```python
from build123d import *

# Parameters (mm, degrees)
SKETCH1_W            = 43.08
SKETCH1_H            = 16.08
SKETCH1_W_2          = 38
SKETCH1_H_2          = 11
BOSS_EXTRUDE1_DEPTH  = 57.785
SKETCH1_2_W          = 43.08
SKETCH1_2_H          = 16.08
SKETCH1_2_W_2        = 38
SKETCH1_2_H_2        = 11
BOSS_EXTRUDE2_DEPTH  = 2.54
CUT_EXTRUDE2_DEPTH   = 2.54
SKETCH5_W            = 11.811
SKETCH5_H            = 43.08
BOSS_EXTRUDE8_DEPTH  = 2.54
SKETCH5_6_R          = 1.27
BOSS_EXTRUDE9_DEPTH  = 6.35
SKETCH5_8_R          = 1.896612794
SKETCH5_8_R_2        = 1.27
BOSS_EXTRUDE10_DEPTH = 3.81
SKETCH6_W            = 43.08
SKETCH6_H            = 16.08
BOSS_EXTRUDE11_DEPTH = 3.81
SKETCH7_W            = 43.08
SKETCH7_H            = 2.54
BOSS_EXTRUDE12_DEPTH = 1.778
SKETCH8_W            = 3.81
SKETCH8_H            = 2.54
BOSS_EXTRUDE15_DEPTH = 6.35
SKETCH8_5_W          = 11.938
SKETCH8_5_H          = 2.54
BOSS_EXTRUDE16_DEPTH = 6.35


with BuildPart() as part:
    # Sketch1 → Boss-Extrude1 (new body)
    with BuildSketch(Plane(origin=(0, 0, 0), x_dir=(0, 0, -1), z_dir=(1, 0, 0))):
        Rectangle(SKETCH1_W, SKETCH1_H)
        Rectangle(SKETCH1_W_2, SKETCH1_H_2, mode=Mode.SUBTRACT)
    extrude(amount=-BOSS_EXTRUDE1_DEPTH)

    # Sketch1_2 → Boss-Extrude2 (add)
    # profile 1 of 2: a face of its own
    with BuildSketch(Plane(origin=(0, 0, 0), x_dir=(0, 0, -1), z_dir=(1, 0, 0))):
        Rectangle(SKETCH1_2_W, SKETCH1_2_H)
        Rectangle(SKETCH1_2_W_2, SKETCH1_2_H_2, mode=Mode.SUBTRACT)
    # profile 2 of 2: a face of its own
    with BuildSketch(Plane(origin=(0, 0, 0), x_dir=(0, 0, -1), z_dir=(1, 0, 0))):
        Rectangle(SKETCH1_2_W_2, SKETCH1_2_H_2)
    extrude(amount=BOSS_EXTRUDE2_DEPTH)

    # Sketch3 → Cut-Extrude2 (cut)
    with BuildSketch(Plane(origin=(0, 0, -21.54), x_dir=(-1, 0, 0), z_dir=(0, 0, -1))):
        Polygon((55.245, 2.921), (55.245, -5.5), (57.785, -5.5), (57.785, 2.96), (57.785, 5.5), (55.245, 5.5), align=None)
    extrude(amount=-CUT_EXTRUDE2_DEPTH, mode=Mode.SUBTRACT)

    # Sketch5 → Boss-Extrude8 (add)
    with BuildSketch(Plane(origin=(0, 8.04, 0), x_dir=(1, 0, 0), z_dir=(0, 1, 0))):
        with Locations((-63.6905, 0)):
            Rectangle(SKETCH5_W, SKETCH5_H)
    extrude(amount=-BOSS_EXTRUDE8_DEPTH)

    # Sketch5_6 → Boss-Extrude9 (add)
    with BuildSketch(Plane(origin=(0, 8.04, 0), x_dir=(1, 0, 0), z_dir=(0, 1, 0))):
        with Locations(Location((-67.4497, 14.236700027, 0), (0, 0, 270))):
            Circle(SKETCH5_6_R)
        with Locations(Location((-67.4497, -14.236700027, 0), (0, 0, 270))):
            Circle(SKETCH5_6_R)
        with Locations(Location((0.3937, -14.236700027, 0), (0, 0, 270))):
            Circle(SKETCH5_6_R)
        with Locations(Location((0.3937, 14.236700027, 0), (0, 0, 90))):
            Circle(SKETCH5_6_R)
    extrude(amount=BOSS_EXTRUDE9_DEPTH)

    # Sketch5_8 → Boss-Extrude10 (add)
    # profile 1 of 4: a face of its own
    with BuildSketch(Plane(origin=(0, 8.04, 0), x_dir=(1, 0, 0), z_dir=(0, 1, 0))):
        with Locations(Location((-67.4497, 14.236700027, 0), (0, 0, 90))):
            Circle(SKETCH5_8_R)
        with Locations(Location((-67.4497, 14.236700027, 0), (0, 0, 270))):
            Circle(SKETCH5_8_R_2, mode=Mode.SUBTRACT)
    # profile 2 of 4: a face of its own
    with BuildSketch(Plane(origin=(0, 8.04, 0), x_dir=(1, 0, 0), z_dir=(0, 1, 0))):
        with Locations(Location((-67.4497, -14.236700027, 0), (0, 0, 90))):
            Circle(SKETCH5_8_R)
    # profile 3 of 4: a face of its own
    with BuildSketch(Plane(origin=(0, 8.04, 0), x_dir=(1, 0, 0), z_dir=(0, 1, 0))):
        with Locations(Location((0.3937, -14.236700027, 0), (0, 0, 90))):
            Circle(SKETCH5_8_R)
    # profile 4 of 4: a face of its own
    with BuildSketch(Plane(origin=(0, 8.04, 0), x_dir=(1, 0, 0), z_dir=(0, 1, 0))):
        with Locations(Location((0.3937, 14.236700027, 0), (0, 0, 90))):
            Circle(SKETCH5_8_R)
    extrude(amount=BOSS_EXTRUDE10_DEPTH)

    # Sketch6 → Boss-Extrude11 (add)
    with BuildSketch(Plane(origin=(2.54, 0, 0), x_dir=(0, 0, -1), z_dir=(1, 0, 0))):
        Rectangle(SKETCH6_W, SKETCH6_H)
    extrude(amount=BOSS_EXTRUDE11_DEPTH)

    # Sketch7 → Boss-Extrude12 (add)
    with BuildSketch(Plane.ZY.offset(69.596)):
        with Locations((0, 6.77)):
            Rectangle(SKETCH7_W, SKETCH7_H)
    extrude(amount=BOSS_EXTRUDE12_DEPTH)

    # Sketch8 → Boss-Extrude15 (add)
    with BuildSketch(Plane.ZY.offset(71.374)):
        with Locations((-23.445, 6.77)):
            Rectangle(SKETCH8_W, SKETCH8_H)
    extrude(amount=-BOSS_EXTRUDE15_DEPTH)

    # Sketch8_5 → Boss-Extrude16 (add)
    with BuildSketch(Plane.ZY.offset(71.374)):
        Polygon((-25.35, 5.5), (-25.35, 8.04), (-25.35, 14.82), (-27.89, 14.82), (-27.89, 5.5), (-27.89, -5.5), (-27.89, -8.04), (-25.35, -8.04), (-25.35, -5.5), align=None)
        Polygon((-39.828, -8.04), (-39.828, -5.5), (-39.828, 14.82), (-42.368, 14.82), (-42.368, -8.04), align=None)
        with Locations((-33.859, -6.77)):
            Rectangle(SKETCH8_5_W, SKETCH8_5_H)
    extrude(amount=-BOSS_EXTRUDE16_DEPTH)


solid = part.part
```
Verification items for the finished model (mm, model axes). A direction names the side the tool comes from. Give positions to 0.01 mm unless a question says otherwise; leave off trailing zeros. Order: outer loops, then holes, each group sorted by start corner. A loop starts at its lowest first (then second) coordinate and runs counter-clockwise, first axis right, second up. Notation, with made-up numbers: M 72.25,-7.75 L 104.25,-7.75 A13 cw 104.25,7.25 Z; hole C -1.75,-1 d5. An arc over 180 degrees is marked long. Return JSON: item names as keys, results as strings. Group by question number.
1) Go/stop test with flat-tipped pins: pin 1 Ø2 at (y, z) = (3, -27.5) entering from +X; pin 2 Ø4 at (x, y) = (-21, 4) entering from -Z; pin 3 Ø1.9 at (x, y) = (-69.5, 13) entering from +Z; pin 4 Ø1 at (y, z) = (10, 8.5) entering from -X. Record where each tip stops, or that it passes through.
2) Section check B-B on z = -17.5. Record the cut outline in (x, y) (3 decimals), and give its area (3 significant figures).
3) Section check A-A on y = 0. Record the cut outline in (x, z) (3 decimals).
4) Section check C-C on x = -15.5. Record the cut outline in (y, z).
5) Scan lines: line 1 (X direction, y = 11.75, z = -14.5); line 2 (Y direction, x = -24.5, z = -5.5); line 3 (Z direction, x = -9, y = 0.75). Record each from-to range of solid material in increasing order.
6) Mould release check, pull along X, two halves, no side actions. Record for faces 1 (the face through (-66.38, 13.1, 14.92)), 2 (the face through (-29, 0, -21.54)), 3 (the face through (6.35, 0, 0)): pulls with the +X half, pulls with the -X half, needs draft (parallel to the pull), parting line crosses it, or undercut.
7) Access from +Z, -Z, +X, -X, +Y, -Y to the whole of each face (thin tool, end or side, straight path). Record for faces 4 (the face through (-68, -1, -25.35)), 5 (the face through (-68, -5.5, -34)), 6 (the face through (-0.09, 13.1, 15.41)), 7 (the face through (-28, 0, 19)).
8) Section check D-D on z = -30.5. Record the cut outline in (x, y), and give its area (3 significant figures).
Answer block:
{
 "1": {"pin 1": "stops at x = -65.02", "pin 2": "stops at z = -21.54", "pin 3": "stops at z = 14.87", "pin 4": "passes through"},
 "2": {"outline": "M -71.374,5.5 L 0,5.5 L 0,-5.5 L -57.785,-5.5 L -57.785,-8.04 L 6.35,-8.04 L 6.35,8.04 L -71.374,8.04 Z", "area": "430 mm^2"},
 "3": {"outline": "M -71.374,-42.368 L -65.024,-42.368 L -65.024,-39.828 L -71.374,-39.828 Z; M -71.374,-27.89 L -65.024,-27.89 L -65.024,-25.35 L -71.374,-25.35 Z; M -57.785,19 L 0,19 L 0,-19 L -55.245,-19 L -55.245,-21.54 L 6.35,-21.54 L 6.35,21.54 L -57.785,21.54 Z"},
 "4": {"outline": "M -8.04,-21.54 L 8.04,-21.54 L 8.04,21.54 L -8.04,21.54 Z; hole M -5.5,-19 L 5.5,-19 L 5.5,19 L -5.5,19 Z"},
 "5": {"line 1": "x = -69.33 to -65.57, -1.48 to 2.27", "line 2": "y = -8.04 to -5.5, 5.5 to 8.04", "line 3": "z = -21.54 to -19, 19 to 21.54"},
 "6": {"face 1": "undercut", "face 2": "needs draft", "face 3": "pulls with the +X half"},
 "7": {"face 4": "+Z, +X, -X, -Y", "face 5": "+X, -X, +Y", "face 6": "+Y", "face 7": "-X"},
 "8": {"outline": "M -71.37,-8.04 L -65.02,-8.04 L -65.02,-5.5 L -71.37,-5.5 Z", "area": "16.1 mm^2"}
}
